Design review of the part built by this model. Coordinates are the model's own, in mm. Face numbers are marked on the shaded views. A direction names the side the tool comes from. Coordinates: 2 decimals unless noted, no trailing zeros. Write each loop counter-clockwise with the first axis right and the second up, starting at its lowest first coordinate (ties: lowest second). Pieces come first, ordered by that corner, then holes. Notation, with made-up numbers: M 84.5,-39 L 95.5,-39 A18 cw 95.5,-23 Z; hole C 71,61.25 d4. An arc over 180 degrees is marked long. Return JSON: item names as keys, results as strings. Group by question number.
```python
from build123d import *

# Parameters (mm, degrees)
PLASTIC_DEPTH   = 2.54
CONTACT_DEPTH   = 0.3
CHAMFER1_SIZE   = 0.1
LPATTERN1_COUNT = 6
LPATTERN1_PITCH = 2.54


with BuildPart() as part:
    # Sketch1 → Plastic (new body)
    with BuildSketch(Plane(origin=(0, 0, 0), x_dir=(0, 0, -1), z_dir=(1, 0, 0))):
        Polygon((-2.04, 1.27), (-0.5, 1.27), (0, 0.77), (0, -0.77), (-0.5, -1.27), (-2.04, -1.27), (-2.54, -0.77), (-2.54, 0.77), align=None)
    extrude(amount=PLASTIC_DEPTH)

    # Sketch2 → Contact (add, symmetric)
    with BuildSketch(Plane(origin=(0, 0, 0), x_dir=(1, 0, 0), z_dir=(0, 1, 0))):
        with BuildLine():
            Line((-1.86, 3.36), (-1.86, -0.67))
            ThreePointArc((-1.86, -0.67), (-1.596396103, -1.306396103), (-0.96, -1.57))
            Line((-0.96, -1.57), (8.9, -1.57))
            Line((8.9, -1.57), (8.9, -0.97))
            Line((8.9, -0.97), (-0.96, -0.97))
            ThreePointArc((-0.96, -0.97), (-1.172132034, -0.882132034), (-1.26, -0.67))
            Line((-1.26, -0.67), (-1.26, 3.36))
            Line((-1.26, 3.36), (-1.86, 3.36))
        make_face()
    extrude(amount=CONTACT_DEPTH, both=True)

    # Chamfer1
    chamfer1_edges = [part.edges().sort_by_distance(p)[0] for p in [
        (8.9, 0, 0.97),
        (8.9, 0.3, 1.27),
        (-1.56, -0.3, -3.36),
        (-1.26, 0, -3.36),
        (-1.86, 0, -3.36),
        (8.9, -0.3, 1.27),
        (8.9, 0, 1.57),
        (-1.56, 0.3, -3.36),
    ]]
    chamfer(chamfer1_edges, length=CHAMFER1_SIZE)

    # LPattern1: part ×6


with BuildPart() as part_1:
    add(part.part)
    with Locations(*[(0, i * LPATTERN1_PITCH, 0) for i in range(1, LPATTERN1_COUNT)]):
        add(part.part)


solid = part_1.part
```
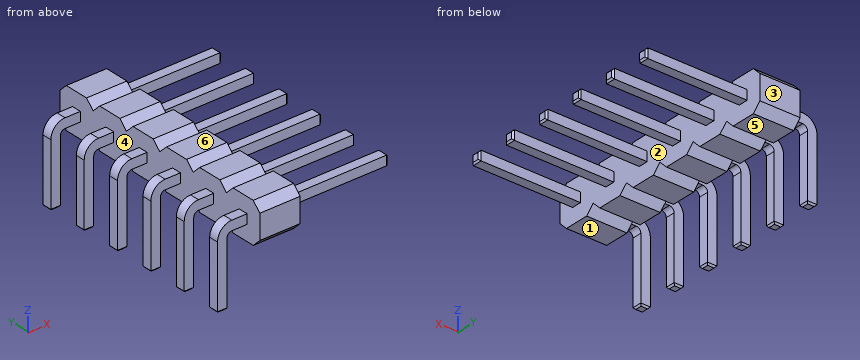
Item 1: Machinability: for the marked faces 5 and 6, which of the approach directions +Z, -Z, +X, -X, +Y, -Y give a long, thin tool a straight path to every point of the face, cutting with its end or side? Answer none if there is none.
Item 2: For line 1 (Y direction, x = -0.25, z = 1.3); line 2 (Z direction, x = 3.5, y = 2.5); line 3 (X direction, y = 7, z = 1.9), list the stretches that pass through material, from the lowest coordinate up.
Item 3: Add section B-B (x = 5.75). Write out the cut boundary in (y, z), plus the area to 3 significant figures.
Item 4: The part is to be moulded in two halves that separate along Y. For the marked faces 1, 2, 3 and 4, say which applies: pulls with the +Y half, pulls with the -Y half, needs draft (parallel to the pull), parting line crosses it, or undercut.
Item 5: Add section A-A (z = -2.2). Write out the cut boundary in (x, y), plus the area to 3 significant figures.
Item 6: Add section C-C (y = 0). Write out the cut boundary in (x, z).
Item 7: For pin 1 (0.5 mm diameter, centred on x = 1, y = 3, fed in from -Z); pin 2 (3 mm diameter, centred on x = 5, y = 1.5, fed in from +Z); pin 3 (0.7 mm diameter, centred on x = -0.5, y = 2.5, fed in from -Z), all flat-tipped, find the tip position at first contact; note any pin that passes through.
Item 8: Add section D-D (y = 3.5). Write out the cut boundary in (x, z).
Geometry check:
{
 "1": {"face 5": "-Z, +X, +Y, -Y", "face 6": "+Z, +X, -X, +Y, -Y"},
 "2": {"line 1": "-0.3 to 0.3, 2.24 to 2.84, 4.78 to 5.38, 7.32 to 7.92, 9.86 to 10.46, 12.4 to 13", "line 2": "0.97 to 1.57", "line 3": "0 to 2.54"},
 "3": {"outline": "M -0.3,0.97 L 0.3,0.97 L 0.3,1.57 L -0.3,1.57 Z; M 2.24,0.97 L 2.84,0.97 L 2.84,1.57 L 2.24,1.57 Z; M 4.78,0.97 L 5.38,0.97 L 5.38,1.57 L 4.78,1.57 Z; M 7.32,0.97 L 7.92,0.97 L 7.92,1.57 L 7.32,1.57 Z; M 9.86,0.97 L 10.46,0.97 L 10.46,1.57 L 9.86,1.57 Z; M 12.4,0.97 L 13,0.97 L 13,1.57 L 12.4,1.57 Z", "area": "2.16 mm^2"},
 "4": {"face 1": "needs draft", "face 2": "undercut", "face 3": "pulls with the +Y half", "face 4": "undercut"},
 "5": {"outline": "M -1.86,-0.3 L -1.26,-0.3 L -1.26,0.3 L -1.86,0.3 Z; M -1.86,2.24 L -1.26,2.24 L -1.26,2.84 L -1.86,2.84 Z; M -1.86,4.78 L -1.26,4.78 L -1.26,5.38 L -1.86,5.38 Z; M -1.86,7.32 L -1.26,7.32 L -1.26,7.92 L -1.86,7.92 Z; M -1.86,9.86 L -1.26,9.86 L -1.26,10.46 L -1.86,10.46 Z; M -1.86,12.4 L -1.26,12.4 L -1.26,13 L -1.86,13 Z", "area": "2.16 mm^2"},
 "6": {"outline": "M -1.86,-3.26 L -1.76,-3.36 L -1.36,-3.36 L -1.26,-3.26 L -1.26,0.67 A0.3 cw -0.96,0.97 L 0,0.97 L 0,0 L 2.54,0 L 2.54,0.97 L 8.8,0.97 L 8.9,1.07 L 8.9,1.47 L 8.8,1.57 L 2.54,1.57 L 2.54,2.54 L 0,2.54 L 0,1.57 L -0.96,1.57 A0.9 ccw -1.86,0.67 Z"},
 "7": {"pin 1": "z = 0", "pin 2": "z = 1.57", "pin 3": "z = 0.97"},
 "8": {"outline": "M 0,0.19 L 2.54,0.19 L 2.54,2.35 L 0,2.35 Z"}
}
